Work out the finished part from the listing and answer in its coordinate system (mm). Face numbers are marked on the shaded views. Round coordinates to 2 decimals unless told otherwise and drop trailing zeros. Order: outer loops, then holes, each group sorted by start corner. A loop starts at its lowest first (then second) coordinate and runs counter-clockwise, first axis right, second up. Notation, with made-up numbers: (31, -6) - (41, -6) arc R16 cw to (41, 15) - close; hole circle Ø5 at (43, 56.25). An arc over 180 degrees is marked (long way). Answer in a Markdown table with one row per item.
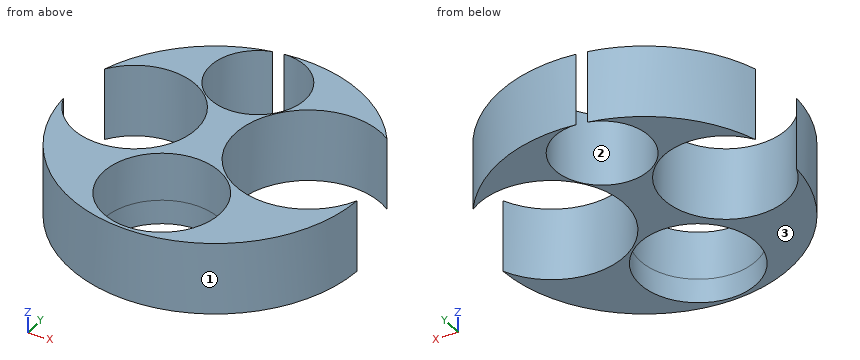
from build123d import *

# Parameters (mm, degrees)
F0_R     = 76.1923930789
F1_DEPTH = 12.7
F2_R     = 30.5006565041
F2_R_2   = 1.4862391827
F3_DEPTH = 12.701
F4_DEPTH = 25.4
F5_DEPTH = 25.4
F6_DEPTH = 25.4
F7_DEPTH = 25.4


with BuildPart() as f1:
    # F0 (on Top) → F1 (new body)
    with BuildSketch(Plane.XY):
        Circle(F0_R)
    extrude(amount=F1_DEPTH)

    # F2 (on face) → F3 (cut, through all)
    with BuildSketch(Plane.XY.offset(12.7)):
        with Locations((-1.4862391827, -43.8670478761)):
            Circle(F2_R)
        with Locations((0, -43.8670478761)):
            Circle(F2_R_2, mode=Mode.SUBTRACT)
        with BuildLine():
            ThreePointArc((76.1923930789, 0), (72.8249793386, 22.4009630914), (63.0203918555, 42.8218515884))
            ThreePointArc((63.0203918555, 42.8218515884), (4.4295199426, 1.2009612876), (76.0198799285, -5.1243164166))
            ThreePointArc((76.0198799285, -5.1243164166), (76.1492525781, -2.5636097365), (76.1923930789, 0))
        make_face()
        with BuildLine():
            ThreePointArc((16.6140991318, 50.8624613285), (8.8970664681, 68.830007636), (-9.4466365709, 75.6045092609))
            ThreePointArc((-9.4466365709, 75.6045092609), (-12.0713018803, 75.2300766582), (-14.6813511871, 74.7645550405))
            ThreePointArc((-14.6813511871, 74.7645550405), (-23.1993361612, 31.1729000429), (16.6140991318, 50.8624613285))
        make_face()
        with BuildLine():
            ThreePointArc((-71.8429908792, 25.374503436), (-75.3423273306, 11.349646492), (-76.1299647651, -3.0837036101))
            ThreePointArc((-76.1299647651, -3.0837036101), (-40.4419002943, -24.9844594479), (-13.2413656339, 6.8496726453))
            ThreePointArc((-13.2413656339, 6.8496726453), (-35.7559759242, 37.5796247979), (-71.8429908792, 25.374503436))
        make_face()
        with BuildLine():
            ThreePointArc((-14.6813511871, 74.7645550405), (-12.0713018803, 75.2300766582), (-9.4466365709, 75.6045092609))
            ThreePointArc((-9.4466365709, 75.6045092609), (-12.0865262133, 75.3249568749), (-14.6813511871, 74.7645550405))
        make_face()
        with BuildLine():
            ThreePointArc((-71.8429908792, 25.374503436), (-77.33938953, 11.6504860173), (-76.1299647651, -3.0837036101))
            ThreePointArc((-76.1299647651, -3.0837036101), (-75.3423273306, 11.349646492), (-71.8429908792, 25.374503436))
        make_face()
        with BuildLine():
            ThreePointArc((76.0198799285, -5.1243164166), (78.7566482722, 2.8459379332), (79.6838716591, 11.2218027934))
            ThreePointArc((79.6838716591, 11.2218027934), (75.2627955479, 29.0840160032), (63.0203918555, 42.8218515884))
            ThreePointArc((63.0203918555, 42.8218515884), (72.8249793386, 22.4009630914), (76.1923930789, 0))
            ThreePointArc((76.1923930789, 0), (76.1492525781, -2.5636097365), (76.0198799285, -5.1243164166))
        make_face()
    extrude(amount=-F3_DEPTH, mode=Mode.SUBTRACT)

    # F4 (add): a face of the model
    f4_faces = [f1.faces().sort_by_distance(p)[0] for p in [
        (-2.154905566, -6.975298751, 12.7),
    ]]
    extrude(f4_faces, amount=F4_DEPTH)

    # F5 (cut): a face of the model
    f5_faces = [f1.faces().sort_by_distance(p)[0] for p in [
        (-2.154905566, -6.975298751, 38.1),
    ]]
    extrude(f5_faces, amount=-F5_DEPTH, mode=Mode.SUBTRACT)

    # F6 (cut): a face of the model
    f6_faces = [f1.faces().sort_by_distance(p)[0] for p in [
        (0, -43.8670478761, 12.7),
    ]]
    extrude(f6_faces, amount=-F6_DEPTH, mode=Mode.SUBTRACT)

    # F7 (add): a face of the model
    f7_faces = [f1.faces().sort_by_distance(p)[0] for p in [
        (-2.154905566, -6.975298751, 12.7),
    ]]
    extrude(f7_faces, amount=F7_DEPTH)


solid = f1.part
1) Each of these flat-tipped pins is pushed along its axis until it touches: pin 1 (12 mm diameter, centred on x = 2.5, z = 34.5, fed in from -Y); pin 2 (12 mm diameter, centred on x = 39.5, z = 15, fed in from +Y); pin 3 (3 mm diameter, centred on y = -36, z = 31, fed in from -X). Where does it stop, or does it pass through?
Filled in:
| item | result |
|---|---|
| pin 1 | stops at y = -76.19 |
| pin 2 | stops at y = 68.43 |
| pin 3 | stops at x = -67.93 |
2) Find section D-D, the plane z = 35. Give the vertices of the cut face in (x, y).
Filled in:
| item | result |
|---|---|
| outline | (-76.13, -3.08) arc R76.19 ccw to (76.02, -5.12) arc R38.29 cw (long way) to (63.02, 42.82) arc R76.19 ccw to (-9.45, 75.6) arc R24.78 cw (long way) to (-14.68, 74.76) arc R76.19 ccw to (-71.84, 25.37) arc R32.23 cw (long way) to start; hole circle Ø61 at (-1.49, -43.87) |
3) Find section C-C, the plane x = 0. Give the vertices of the cut face in (y, z).
Filled in:
| item | result |
|---|---|
| outline | (-76.19, 0) - (-74.33, 0) - (-74.33, 38.1) - (-76.19, 38.1) - close; (-13.4, 0) - (27.47, 0) - (27.47, 38.1) - (-13.4, 38.1) - close; (74.26, 0) - (76.19, 0) - (76.19, 38.1) - (74.26, 38.1) - close |
4) The mould has two halves that part along X. Classify the marked faces 1, 2 and 3: released by +X, released by -X, zero draft, split by the parting line, or undercut.
Filled in:
| item | result |
|---|---|
| face 1 | split by the parting line |
| face 2 | undercut |
| face 3 | zero draft |
5) Find section B-B, the plane x = 38.5. Give the vertices of the cut face in (y, z).
Filled in:
| item | result |
|---|---|
| outline | (-65.75, 0) - (-26.96, 0) - (-26.96, 38.1) - (-65.75, 38.1) - close; (49.41, 0) - (65.75, 0) - (65.75, 38.1) - (49.41, 38.1) - close |
6) Find the intervals of material crossed by probe 1 along Y at (x, z) = (23, 2.5); probe 2 along X at (y, z) = (45, 9); probe 3 along Y at (x, z) = (-26, 9), in increasing order. Write a range as from..to.
Filled in:
| item | result |
|---|---|
| probe 1 | y = -72.64..-62.05, -25.68..-22.37, 44.81..72.64 |
| probe 2 | x = -61.48..-32.23, 15.91..23.35, 59.43..61.48 |
| probe 3 | y = -71.62..-62.02, -25.72..-18.83, 32.53..33.67, 68.06..71.62 |
7) Find section A-A, the plane y = -48. Give the vertices of the cut face in (x, z).
Filled in:
| item | result |
|---|---|
| outline | (-59.17, 0) - (-31.71, 0) - (-31.71, 38.1) - (-59.17, 38.1) - close; (28.73, 0) - (59.17, 0) - (59.17, 38.1) - (28.73, 38.1) - close |
